Source: CAD feature listing. Evaluate the final solid. Frame: model axes, mm. A direction names the side the tool comes from. Coordinates: 2 decimals unless noted, no trailing zeros. Order: outer loops, then holes, each group sorted by start corner. A loop starts at its lowest first (then second) coordinate and runs counter-clockwise, first axis right, second up. Notation, with made-up numbers: (21, 89) -> (62, 89) arc R31 cw to (62, 122) -> close; hole circle Ø8 at (8, -35). An arc over 180 degrees is marked (long way). Write item = value, one per line. Start each with the question number.
Item 1: Section query B-B (z = 2). Output: boundary loops of the cut face in (x, y), then the cut area to 4 significant figures.
Item 2: Set-up query: faces 1 (the flat face through (0, -6, 0)), 2 (the flat face through (0, -3.25, 0)), 3 (the cylindrical face through (-1.57, -4.64, 0.45)). Return all of +Z, -Z, +X, -X, +Y, -Y with unobstructed straight access to the full face (end or side cutting, diameter ignored); none if empty.
Item 3: Section query D-D (x = 3). Output: boundary loops of the cut face in (y, z).
Item 4: Section query C-C (x = -1). Output: boundary loops of the cut face in (y, z), then the cut area to 3 significant figures.
Item 5: Section query A-A (y = -1.5). Output: boundary loops of the cut face in (x, z).
Item 6: Ray query, line 1 along Y through (x, z) = (-1.5, 1.2); line 2 along X through (y, z) = (-2, -1.3); line 3 along Z through (x, y) = (-3, -3.95). Return the intervals inside material, ascending. Write a range as [from, to].
Item 7: Mould query, pull axis X, two halves, no side actions, for faces 4 (the flat face through (0, 6, 0)), 5 (the cylindrical face through (4.386, -4.644, -0.575)), 6 (the flat face through (-7.5, 0, 0)), 7 (the flat face through (7.5, 0, 0)). Classes: released by +X, released by -X, zero draft, split by the parting line, or undercut.
```python
from build123d import *

# Parameters (mm, degrees)
SKETCH_1_W          = 15
SKETCH_1_H          = 12
EXTRUDE_1_DEPTH     = 2.5
SKETCH_2_W          = 9
SKETCH_2_H          = 6.5
CUT_EXTRUDE_1_DEPTH = 6
CUT_EXTRUDE_2_REACH = 14
SKETCH_3_R          = 1.5


with BuildPart() as part:
    # 草圖1 → 填料-伸長1 (new body, symmetric)
    with BuildSketch(Plane.XY):
        Rectangle(SKETCH_1_W, SKETCH_1_H)
    extrude(amount=EXTRUDE_1_DEPTH, both=True)

    # 草圖2 → 除料-伸長1 (cut, through all)
    with BuildSketch(Plane.XY.offset(2.5)):
        Rectangle(SKETCH_2_W, SKETCH_2_H)
    extrude(amount=-CUT_EXTRUDE_1_DEPTH, mode=Mode.SUBTRACT)

    # 草圖3 → 除料-伸長2 (cut, up to next)
    with BuildSketch(Plane.XZ.offset(6), mode=Mode.PRIVATE) as cut_extrude_2_sk1:
        with Locations((-3, 0)):
            Circle(SKETCH_3_R)
    cut_extrude_2_tool1 = extrude(cut_extrude_2_sk1.sketch, amount=-CUT_EXTRUDE_2_REACH, mode=Mode.PRIVATE) & part.part
    add(cut_extrude_2_tool1.solids().sort_by_distance((-3, -6, 0))[0], mode=Mode.SUBTRACT)
    # 草圖3 → 除料-伸長2 (cut, up to next)
    with BuildSketch(Plane.XZ.offset(6), mode=Mode.PRIVATE) as cut_extrude_2_sk2:
        with Locations((3, 0)):
            Circle(SKETCH_3_R)
    cut_extrude_2_tool2 = extrude(cut_extrude_2_sk2.sketch, amount=-CUT_EXTRUDE_2_REACH, mode=Mode.PRIVATE) & part.part
    add(cut_extrude_2_tool2.solids().sort_by_distance((3, -6, 0))[0], mode=Mode.SUBTRACT)


solid = part.part
```
Computed:
q1.outline = (-7.5, -6) -> (7.5, -6) -> (7.5, 6) -> (-7.5, 6) -> close; hole (-4.5, -3.25) -> (4.5, -3.25) -> (4.5, 3.25) -> (-4.5, 3.25) -> close
q1.area = 121.5 mm^2
q2.face_1 = +Z, -Z, +X, -X, -Y
q2.face_2 = +Z, -Z
q2.face_3 = -Y
q3.outline = (-6, -2.5) -> (-3.25, -2.5) -> (-3.25, -1.5) -> (-6, -1.5) -> close; (-6, 1.5) -> (-3.25, 1.5) -> (-3.25, 2.5) -> (-6, 2.5) -> close; (3.25, -2.5) -> (6, -2.5) -> (6, 2.5) -> (3.25, 2.5) -> close
q4.outline = (-6, -2.5) -> (-3.25, -2.5) -> (-3.25, 2.5) -> (-6, 2.5) -> close; (3.25, -2.5) -> (6, -2.5) -> (6, 2.5) -> (3.25, 2.5) -> close
q4.area = 27.5 mm^2
q5.outline = (-7.5, -2.5) -> (-4.5, -2.5) -> (-4.5, 2.5) -> (-7.5, 2.5) -> close; (4.5, -2.5) -> (7.5, -2.5) -> (7.5, 2.5) -> (4.5, 2.5) -> close
q6.line_1 = [-6, -3.25], [3.25, 6]
q6.line_2 = [-7.5, -4.5], [4.5, 7.5]
q6.line_3 = [-2.5, -1.5], [1.5, 2.5]
q7.face_4 = zero draft
q7.face_5 = undercut
q7.face_6 = released by -X
q7.face_7 = released by +X
